```python
from build123d import *

# Parameters (mm, degrees)
SKETCH_W        = 100
SKETCH_H        = 100
PAD_DEPTH       = 20
SKETCH001_W     = 48
SKETCH001_H     = 48
POCKET_DEPTH    = 10
SKETCH002_R     = 10
POCKET001_DEPTH = 15
PAD001_DEPTH    = 5
SKETCH004_W     = 15
SKETCH004_H     = 15
PAD002_DEPTH    = 5
SKETCH005_R     = 6
POCKET002_DEPTH = 10


with BuildPart() as part:
    # Sketch → Pad (new body)
    with BuildSketch(Plane.XY):
        Rectangle(SKETCH_W, SKETCH_H)
    extrude(amount=-PAD_DEPTH)

    # Sketch001 (on Face5 of Pad) → Pocket (cut)
    with BuildSketch(Plane.XY):
        with Locations((0, 25)):
            Rectangle(SKETCH001_W, SKETCH001_H)
        with Locations((0, -25)):
            Rectangle(SKETCH001_W, SKETCH001_H)
    extrude(amount=-POCKET_DEPTH, mode=Mode.SUBTRACT)

    # Sketch002 (on Face4 of Pocket) → Pocket001 (cut)
    with BuildSketch(Plane.XY):
        with Locations((-24, 30)):
            Circle(SKETCH002_R)
        with Locations((-38, 0)):
            Circle(SKETCH002_R)
        with Locations((0, 38)):
            Circle(SKETCH002_R)
        with Locations((24, 30)):
            Circle(SKETCH002_R)
    extrude(amount=-POCKET001_DEPTH, mode=Mode.SUBTRACT)

    # Sketch003 → Pad001 (join)
    with BuildSketch(Plane.XY.offset(-10)):
        Polygon((12.990381, -32.5), (12.990381, -17.5), (0, -10), (-12.990381, -17.5), (-12.990381, -32.5), (0, -40), align=None)
    extrude(amount=PAD001_DEPTH)

    # Sketch004 (on Face33 of Pad001) → Pad002 (join)
    with BuildSketch(Plane.XY.offset(-5)):
        with Locations((0, -25)):
            Rectangle(SKETCH004_W, SKETCH004_H)
    extrude(amount=PAD002_DEPTH)

    # Sketch005 (on Face38 of Pad002) → Pocket002 (cut)
    with BuildSketch(Plane.XY):
        with Locations((0, -25)):
            Circle(SKETCH005_R)
    extrude(amount=-POCKET002_DEPTH, mode=Mode.SUBTRACT)


solid = part.part
```
Can you work these out from the model? Positions are in its coordinate system, mm. A direction names the side the tool comes from. Give positions to 0.01 mm unless a question says otherwise; leave off trailing zeros. Loops run counter-clockwise (first coordinate to the right, second up) from the corner with the lowest first, then second, coordinate; pieces in that order, holes last. Notation, with made-up numbers: M 3.25,50.5 L 45.25,50.5 A5 ccw 45.25,56.5 Z; hole C 16,47.25 d10. An arc over 180 degrees is marked long. Use CSV: the item, a comma, the result in double quotes. Start each with the question number.
1. Imagine slicing it at C-C, the plane y = 30. Write out the boundary of the cut face in (x, z).
2. On a 3-axis mill with a long thin cutter (end or side, diameter ignored), from which of +Z, -Z, +X, -X, +Y, -Y can I reach the whole of each face in a straight line? I mean faces 1 (the face through (0, 38, -15)), 2 (the face through (-1, 50, -10)). Say none if no direction works.
3. Imagine slicing it at A-A, the plane z = -7.75. Write out the boundary of the cut face in (x, y), plus the area to 3 significant figures.
4. If I drill on L1, parallel to Y at x = 0, z = -2.75; L2, parallel to Y at x = -32, z = -13; L3, parallel to X at y = 35.5, z = -14.25, over which ranges is the centre line in solid material (lowest first)?
5. Imagine slicing it at D-D, the plane x = -2.5. Write out the boundary of the cut face in (y, z), plus the area to 3 significant figures.
6. For P1, Ø18, axis at x = 24, y = 30, coming from the +Z side, with a flat end and sliding along its axis, tell me the tip position at first contact or that it passes through.
7. Imagine slicing it at B-B, the plane z = -12.75. Write out the boundary of the cut face in (x, y), plus the area to 3 significant figures.
Response values:
1,outline,"M -50,-20 L 50,-20 L 50,0 L 34,0 L 34,-15 L 14,-15 L 14,-10 L 6,-10 L 6,-15 L -6,-15 L -6,-10 L -14,-10 L -14,-15 L -34,-15 L -34,0 L -50,0 Z"
2,face 1,"+Z"
2,face 2,"+Z, -Z, +X, -X, +Y"
3,outline,"M -50,-50 L 50,-50 L 50,50 L -50,50 Z; M -12.99,-32.5 L 0,-40 L 12.99,-32.5 L 12.99,-17.5 L 0,-10 L -12.99,-17.5 Z; hole C -38,0 d20; hole M -24,-49 L 24,-49 L 24,-1 L -24,-1 Z; hole M -24,1 L 24,1 L 24,20 A10 ccw 24,40 L 24,49 L -24,49 L -24,40 A10 ccw -24,20 Z; hole C 0,-25 d12"
3,area,"5,240 mm^2"
4,L1,"-50 to -49, -32.5 to -31, -19 to -17.5, -1 to 1, 49 to 50"
4,L2,"-50 to -8, 8 to 24, 36 to 50"
4,L3,"-50 to -32.35, -15.65 to -9.68, 9.68 to 15.65, 32.35 to 50"
5,outline,"M -50,-20 L 50,-20 L 50,0 L 49,0 L 49,-10 L 47.68,-10 L 47.68,-15 L 28.32,-15 L 28.32,-10 L 1,-10 L 1,0 L -1,0 L -1,-10 L -11.44,-10 L -11.44,-5 L -17.5,-5 L -17.5,0 L -19.55,0 L -19.55,-10 L -30.45,-10 L -30.45,0 L -32.5,0 L -32.5,-5 L -38.56,-5 L -38.56,-10 L -49,-10 L -49,0 L -50,0 Z"
5,area,"1,040 mm^2"
6,P1,"z = -15"
7,outline,"M -50,-50 L 50,-50 L 50,50 L -50,50 Z; hole C -38,0 d20; hole C -24,30 d20; hole C 0,38 d20; hole C 24,30 d20"
7,area,"8,740 mm^2"
